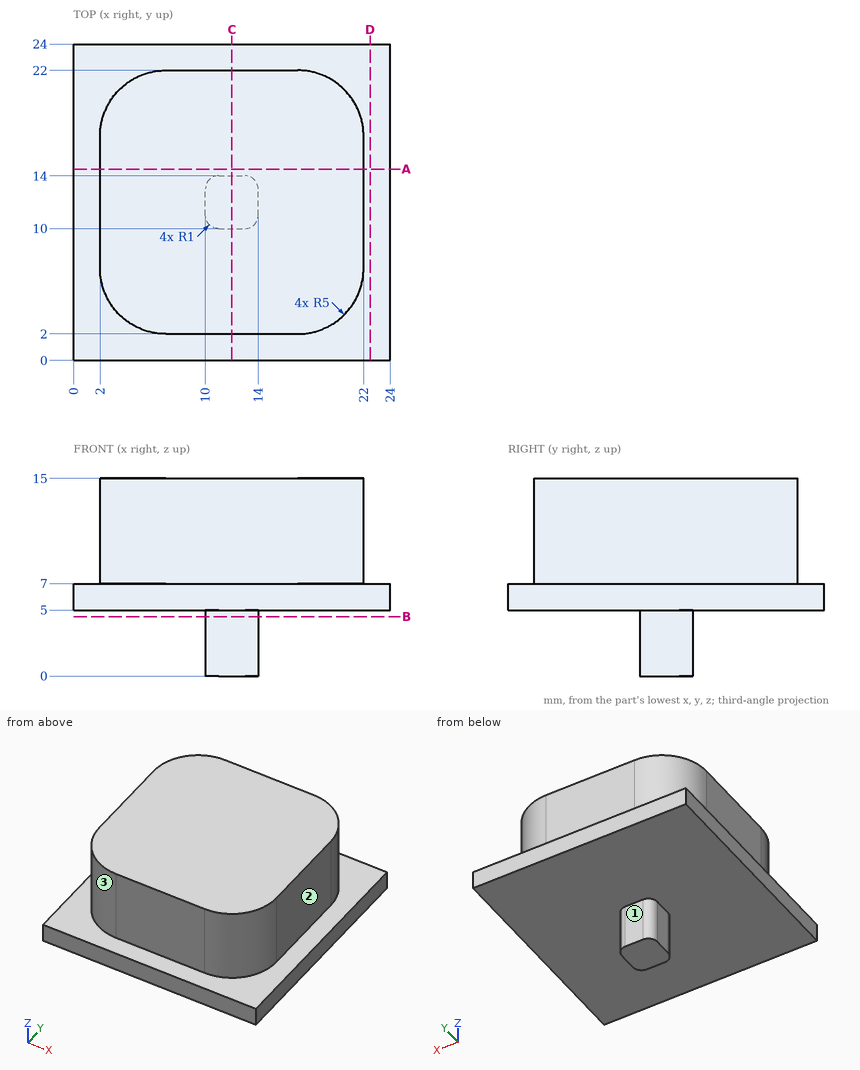
Verification items for this drawing (mm, ordinates from the low corner). A direction names the side the tool comes from. Give positions to 0.01 mm unless a question says otherwise; leave off trailing zeros. Loops run counter-clockwise (first coordinate to the right, second up) from the corner with the lowest first, then second, coordinate; pieces in that order, holes last.
1. Go/stop test with flat-tipped pins: P1, Ø1, axis at y = 4, z = 9, coming from the +X side; P2, Ø2.5, axis at y = 14, z = 9.5, coming from the -X side; P3, Ø2, axis at x = 11.5, z = 1.5, coming from the +Y side. Record where each tip stops, or that it passes through.
Derived:
P1: stops at x = 21.33
P2: stops at x = 2
P3: stops at y = 14
2. Cross-section at A-A on y = 14.5. Record the cut outline in (x, z).
Derived:
outline: (0, 5) - (24, 5) - (24, 7) - (22, 7) - (22, 15) - (2, 15) - (2, 7) - (0, 7) - close
3. Cross-section at B-B on z = 4.5. Record the cut outline in (x, y).
Derived:
outline: (10, 11) arc R1 ccw to (11, 10) - (13, 10) arc R1 ccw to (14, 11) - (14, 13) arc R1 ccw to (13, 14) - (11, 14) arc R1 ccw to (10, 13) - close
4. Material ranges on probe 1 along X at (y, z) = (16.5, 12); probe 2 along X at (y, z) = (13, 3.5); probe 3 along Z at (x, y) = (14.75, 16.5), recorded low to high.
Derived:
probe 1: x = 2 to 22
probe 2: x = 10 to 14
probe 3: z = 5 to 15
5. Cross-section at D-D on x = 22.5. Record the cut outline in (y, z), and give its area (3 significant figures).
Derived:
outline: (0, 5) - (24, 5) - (24, 7) - (0, 7) - close
area: 48.0 mm2
6. Tool access check on the marked faces 1, 2 and 3. Record the directions out of +Z, -Z, +X, -X, +Y, -Y that give a thin tool (end or side, any length) a straight path to the whole face; none if there is none.
Derived:
face 1: -Z, +X, -X, +Y
face 2: +Z, +X, +Y, -Y
face 3: +Z, -X, -Y
7. Cross-section at C-C on x = 12. Record the cut outline in (y, z), and give its area (3 significant figures).
Derived:
outline: (0, 5) - (10, 5) - (10, 0) - (14, 0) - (14, 5) - (24, 5) - (24, 7) - (22, 7) - (22, 15) - (2, 15) - (2, 7) - (0, 7) - close
area: 228 mm2
